Part print with two shaded views. Sizes in mm from the minimum x, y, z corner. Round coordinates to 2 decimals unless told otherwise and drop trailing zeros. Order: outer loops, then holes, each group sorted by start corner. A loop starts at its lowest first (then second) coordinate and runs counter-clockwise, first axis right, second up. Notation, with made-up numbers: M 11,39 L 44,39 A20 ccw 44,53 Z; hole C 34,-19.75 d7. An arc over 180 degrees is marked long. Put each result on its own line as item: value.
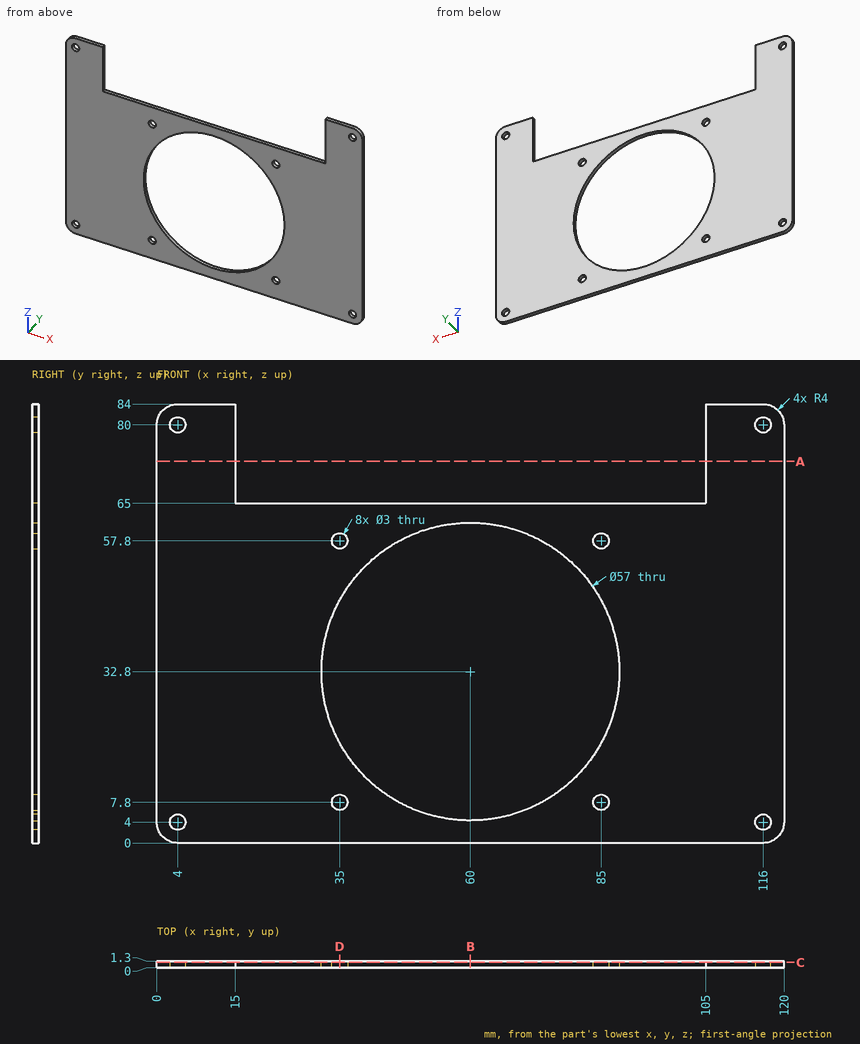
Item 1: Band-saw the part on B-B on x = 60. Give the cut face in (y, z), and give its area (3 significant figures).
Answers below:
outline: M 0,0 L 1.3,0 L 1.3,4.3 L 0,4.3 Z; M 0,61.3 L 1.3,61.3 L 1.3,65 L 0,65 Z
area: 10.4 mm²
Item 2: Band-saw the part on A-A on z = 73. Give the cut face in (x, y), and give its area (3 significant figures).
Answers below:
outline: M 0,0 L 15,0 L 15,1.3 L 0,1.3 Z; M 105,0 L 120,0 L 120,1.3 L 105,1.3 Z
area: 39.0 mm²
Item 3: Pin check, flat tip, straight feed: P1, Ø0.6, axis at x = 70, y = 0.5, coming from the +Z side. Stop position of the tip, or through.
Answers below:
P1: z = 65
Item 4: Band-saw the part on D-D on x = 35. Give the cut face in (y, z), and give its area (3 significant figures).
Answers below:
outline: M 0,0 L 1.3,0 L 1.3,6.3 L 0,6.3 Z; M 0,9.3 L 1.3,9.3 L 1.3,19.12 L 0,19.12 Z; M 0,46.48 L 1.3,46.48 L 1.3,56.3 L 0,56.3 Z; M 0,59.3 L 1.3,59.3 L 1.3,65 L 0,65 Z
area: 41.1 mm²
Item 5: Band-saw the part on C-C on y = 1.05. State how many separate pieces and enclosed holes the cut face has, and give its area (3 significant figures).
Answers below:
separate pieces: 1
enclosed holes: 9
area: 5,750 mm²
Item 6: Probe line 1 along Z through (x, y) = (116, 0.45); line 2 along X through (y, z) = (0.9, 80); line 3 along X through (y, z) = (1, 4). List the from-to ranges inside material, lowest first. Write a range as [from, to].
Answers below:
line 1: [0, 2.5], [5.5, 78.5], [81.5, 84]
line 2: [0, 2.5], [5.5, 15], [105, 114.5], [117.5, 120]
line 3: [0, 2.5], [5.5, 114.5], [117.5, 120]
